Source: three-view drawing plus pictorial views. Frame: mm from the lowest corner of the part. A direction names the side the tool comes from. Coordinates: 2 decimals unless noted, no trailing zeros. Write each loop counter-clockwise with the first axis right and the second up, starting at its lowest first coordinate (ties: lowest second). Pieces come first, ordered by that corner, then holes. Notation, with made-up numbers: (-25, 45) - (15, 45) arc R4 ccw to (15, 50) - close; hole circle Ø2 at (-1.75, 24). An arc over 180 degrees is marked (long way). Put each result on its own line as item: value. Start each with the question number.
1. Cut plane B-B, the plane z = 5.25. Return loops of the section in (x, y).
2. Access query for the marked faces 5, 6 and 7. Directions: +Z, -Z, +X, -X, +Y, -Y. A direction counts if a zero-diameter tool reaches every point of the face in a straight line with its end or side. Return the directions, or none.
3. Cut plane D-D, the plane y = 4.75. Return loops of the section in (x, z).
4. Cut plane C-C, the plane x = 11.75. Return loops of the section in (y, z), and give its area (3 significant figures).
5. Cut plane A-A, the plane z = 8.5. Return loops of the section in (x, y), and give its area (3 significant figures).
6. Pin query (flat end, axial travel): pin 1 (1.5 mm diameter, centred on y = 6, z = 8.5, fed in from -X); pin 2 (1.6 mm diameter, centred on x = 11, y = 12.5, fed in from -Z); pin 3 (9 mm diameter, centred on x = 14, z = 5, fed in from +Y); pin 4 (0.6 mm diameter, centred on y = 1, z = 14, fed in from -X). Return the tip coordinate at first contact, or that it passes through.
7. Line query: line 1 (Y direction, x = 17.25, z = 8); line 2 (X direction, y = 8.5, z = 2); line 3 (Z direction, x = 10.5, y = 10.5). Output: solid intervals per line, ascending.
8. Pull-direction query (X, two-part tool) for the marked faces 1, 2, 3 and 4; classes: released by +X, released by -X, zero draft, split by the parting line, or undercut.
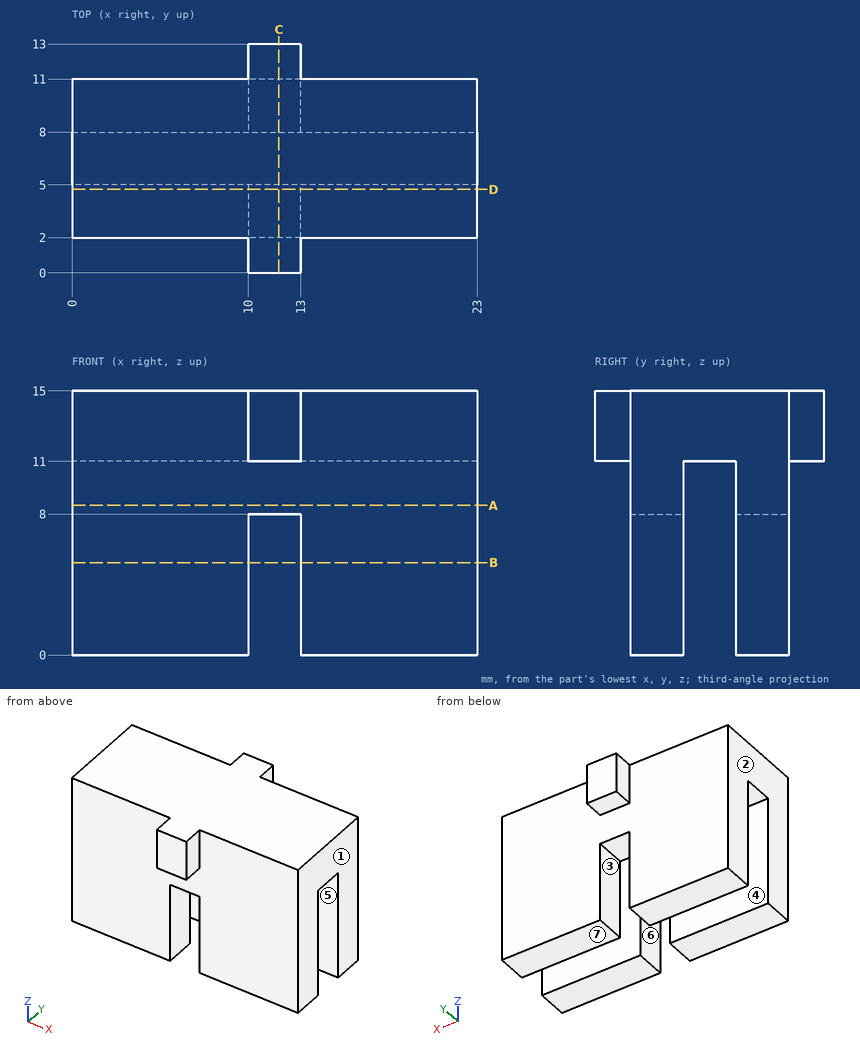
Report:
1. outline: (0, 2) - (10, 2) - (10, 5) - (0, 5) - close; (0, 8) - (10, 8) - (10, 11) - (0, 11) - close; (13, 2) - (23, 2) - (23, 5) - (13, 5) - close; (13, 8) - (23, 8) - (23, 11) - (13, 11) - close
2. face 5: -Z, +X, -X
2. face 6: -Z, +Y, -Y
2. face 7: -Z, +X, -X, +Y, -Y
3. outline: (0, 0) - (10, 0) - (10, 8) - (13, 8) - (13, 0) - (23, 0) - (23, 15) - (0, 15) - close
4. outline: (0, 11) - (2, 11) - (2, 8) - (5, 8) - (5, 11) - (8, 11) - (8, 8) - (11, 8) - (11, 11) - (13, 11) - (13, 15) - (0, 15) - close
4. area: 70.0 mm^2
5. outline: (0, 2) - (23, 2) - (23, 5) - (0, 5) - close; (0, 8) - (23, 8) - (23, 11) - (0, 11) - close
5. area: 138 mm^2
6. pin 1: passes through
6. pin 2: stops at z = 11
6. pin 3: stops at y = 11
6. pin 4: stops at x = 10
7. line 1: y = 2 to 5, 8 to 11
7. line 2: x = 0 to 10, 13 to 23
7. line 3: z = 8 to 15
8. face 1: released by +X
8. face 2: released by -X
8. face 3: undercut
8. face 4: zero draft
